Input: part model. Units: mm. Frame: model coordinates. A direction names the side the tool comes from. Coordinates: 2 decimals unless noted, no trailing zeros. Loops run counter-clockwise (first coordinate to the right, second up) from the corner with the lowest first, then second, coordinate; pieces in that order, holes last.
Autodesk Fusion 360 part; units mm, degrees
sketch "Skizze1" plane through (0, 0, 0) normal (0, 0, 1) x (1, 0, 0)
  circle A0 centre (0, 0) radius 7.8
  circle A1 centre (0, 0) radius 8.8
  line L0 (1.2, -1.7) -> (-1.2, -1.7)
  line L1 (-1.2, -1.7) -> (-1.2, 1.7)
  line L2 (-1.2, 1.7) -> (1.2, 1.7)
  line L3 (1.2, 1.7) -> (1.2, -1.7)
  line L4 (1.2, -1.7) -> (-1.2, 1.7) construction
  line L5 (-1.2, -1.7) -> (1.2, 1.7) construction
  line L6 (4.75, -4.75) -> (-4.75, 4.75) construction
  line L7 (-4.75, -4.75) -> (4.75, 4.75) construction
  circle A2 centre (0, 0) radius 6.9
  line L8 (-1.8, -1.8) -> (1.8, -1.8)
  line L9 (1.8, -1.8) -> (1.8, 1.8)
  line L10 (1.8, 1.8) -> (-1.8, 1.8)
  line L11 (-1.8, 1.8) -> (-1.8, -1.8)
  line L12 (-1.8, -1.8) -> (1.8, 1.8) construction
  line L13 (1.8, -1.8) -> (-1.8, 1.8) construction
  line L14 (-3.5, -3.5) -> (3.5, -3.5)
  line L15 (3.5, -3.5) -> (3.5, 3.5)
  line L16 (3.5, 3.5) -> (-3.5, 3.5)
  line L17 (-3.5, 3.5) -> (-3.5, -3.5)
  line L18 (-3.5, -3.5) -> (3.5, 3.5) construction
  line L19 (3.5, -3.5) -> (-3.5, 3.5) construction
  dimension "d1" = 15.6
  dimension "d2" = 17.6
  dimension "d5" = 2.4
  dimension "d6" = 3.4
  dimension "d17" = 13.8
  dimension "d18" = 3.6
  dimension "d19" = 3.6
  dimension "d20" = 7
  dimension "d21" = 7
extrude "Extrusion1" add sketch "Skizze1" along normal blind 9 contours A0 | L0 L1 L2 L3 | A2 | L8 L9 L10 L11 | L14 L15 L16 L17
extrude "Extrusion2" add sketch "Skizze1" along normal blind 2 contours A1
extrude "Extrusion5" cut sketch "Skizze1" along normal blind 8 contours A2
extrude "Extrusion6" cut sketch "Skizze1" along normal blind 5 contours L14 L15 L16 L17
extrude "Extrusion7" cut sketch "Skizze1" along normal blind 4.5 contours L8 L9 L10 L11
extrude "Extrusion8" cut sketch "Skizze1" along normal blind 7 contours L0 L1 L2 L3
fillet "Abrundung1" radius 1 1 edges at (-7.2722, -2.8206, 9)
Item 1: Section query B-B (x = 0). Output: boundary loops of the cut face in (y, z).
Result:
outline: (-8.8, 0) - (-6.9, 0) - (-6.9, 8) - (-3.5, 8) - (-3.5, 5) - (-1.8, 5) - (-1.8, 4.5) - (-1.7, 4.5) - (-1.7, 7) - (1.7, 7) - (1.7, 4.5) - (1.8, 4.5) - (1.8, 5) - (3.5, 5) - (3.5, 8) - (6.9, 8) - (6.9, 0) - (8.8, 0) - (8.8, 2) - (7.8, 2) - (7.8, 8) arc R1 ccw to (6.8, 9) - (-6.8, 9) arc R1 ccw to (-7.8, 8) - (-7.8, 2) - (-8.8, 2) - close
Item 2: Section query A-A (y = 0). Output: boundary loops of the cut face in (x, z), then the cut area to 3 significant figures.
Result:
outline: (-8.8, 0) - (-6.9, 0) - (-6.9, 8) - (-3.5, 8) - (-3.5, 5) - (-1.8, 5) - (-1.8, 4.5) - (-1.2, 4.5) - (-1.2, 7) - (1.2, 7) - (1.2, 4.5) - (1.8, 4.5) - (1.8, 5) - (3.5, 5) - (3.5, 8) - (6.9, 8) - (6.9, 0) - (8.8, 0) - (8.8, 2) - (7.8, 2) - (7.8, 8) arc R1 ccw to (6.8, 9) - (-6.8, 9) arc R1 ccw to (-7.8, 8) - (-7.8, 2) - (-8.8, 2) - close
area: 50.4 mm2
Item 3: Line query: L1, parallel to Y at x = 0, z = 6; L2, parallel to Y at x = 0, z = 4; L3, parallel to X at y = -0.25, z = 1.75. Output: solid intervals per line, ascending.
Result:
L1: y = -7.8 to -6.9, -3.5 to -1.7, 1.7 to 3.5, 6.9 to 7.8
L2: y = -7.8 to -6.9, 6.9 to 7.8
L3: x = -8.8 to -6.9, 6.9 to 8.8
Item 4: Mould query, pull axis X, two halves, no side actions, for faces 1 (the face through (-1, -8, 2)), 2 (the face through (0, -3.5, 6)), 3 (the face through (8.394, -2.643, 0.986)). Classes: +X half, -X half, draft (parallel to the pull), parting line (faces both ways), or undercut.
Result:
face 1: draft
face 2: undercut
face 3: parting line
Item 5: Reachability of faces 4 (the face through (-5, -5, 0)), 5 (the face through (-5.75, -5.27, 4.96)), 6 (the face through (3.5, 0, 6)) from +Z, -Z, +X, -X, +Y, -Y: full face, straight path, thin tool, end or side. Return the list, or none.
Result:
face 4: -Z, +X, -X, +Y, -Y
face 5: +Z
face 6: -Z
Item 6: Contact query for flat-ended pins moving along their axis: P1, Ø1.9, axis at x = 0.5, z = 6.5, coming from the -Y side; P2, Ø7.5, axis at x = -0.5, y = 0, coming from the -Z side; P3, Ø5, axis at y = 3, z = 3.5, coming from the +X side. Output: stop coordinate, or through.
Result:
P1: stops at y = -7.8
P2: stops at z = 4.5
P3: stops at x = 8.74
